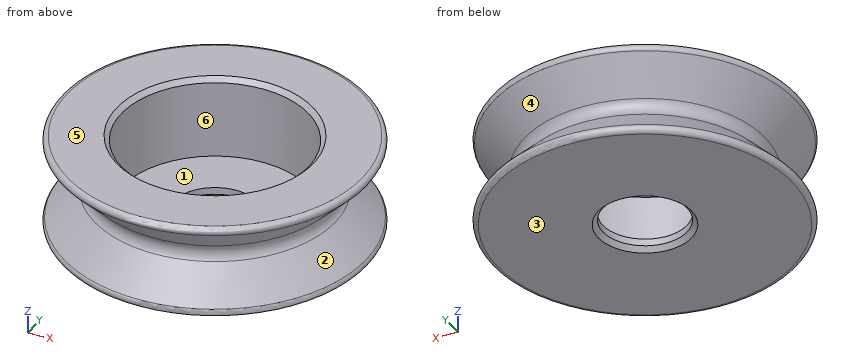
Solid Edge part; units mm, degrees
sketch "Sketch1" plane through (0, 0, 0) normal (0, -1, 0) x (1, 0, 0)
  line L0 (6.7929, 2) -> (1.8, 2)
  line L1 (1.8, 2) -> (1.8, -2)
  line L2 (1.8, -2) -> (6.7929, -2)
  line L3 (6.7929, -2) -> (5.1464, -0.3536)
  line L4 (5.1464, 0.3536) -> (6.7929, 2)
  arc A0 (5.1464, -0.3536) -> (5.1464, 0.3536) centre (5.5, 0) cw
revolve "RevolvedProtrusion1" add sketch "Sketch1" angle 360 about axis through (0, 0, 2) along (0, 0, -1)
fillet "Round1" radius 0.2 2 edges at (-6.7929, 0, 2) (-6.7929, 0, -2)
sketch "Sketch2" plane through (0, 0, 2) normal (0, 0, 1) x (0, 1, 0)
  circle A0 centre (0, 0) radius 4
extrude "VaciadoExtruido_2" cut sketch "Sketch2" against normal blind 3.5
chamfer "Chaflán_1" distance 0.2 angle 45 2 edges at (0, -4, 2) (-1.8, 0, -2)
Part model, mm, in its own coordinate system. Face numbers are marked on the shaded views. A direction names the side the tool comes from. Coordinates: 2 decimals unless noted, no trailing zeros. Order: outer loops, then holes, each group sorted by start corner. A loop starts at its lowest first (then second) coordinate and runs counter-clockwise, first axis right, second up. Notation, with made-up numbers: (20.5, 64) -> (65.5, 64) arc R15 ccw to (65.5, 81) -> close; hole circle Ø1 at (32.25, 45). An arc over 180 degrees is marked (long way). Put each result on its own line as item: value. Start each with the question number.
(1) Mould opens along Z. For the marked faces 1, 2, 3 and 4 say: pulls with the +Z half, pulls with the -Z half, needs draft (parallel to the pull), parting line crosses it, or undercut.
(2) Band-saw the part on C-C (z = 0.2). Give the cut face in (x, y).
(3) Band-saw the part on D-D (z = 1). Give the cut face in (x, y), then the cut area to 3 significant figures.
(4) Probe line 1 along X through (y, z) = (0, 1.15); line 2 along Y through (x, z) = (-0.25, 0.35); line 3 along Y through (x, z) = (-3.5, 1.4). List the from-to ranges inside material, lowest first. Write a range as [from, to].
(5) Band-saw the part on A-A (x = 0). Give the cut face in (y, z).
(6) Which spindle directions (+Z, -Z, +X, -X, +Y, -Y) get a long thin tool onto all of the face, cutting with end or side? Do the marked faces 5 and 6. Say none if no direction does.
(7) Pin check, flat tips, straight feed: pin 1 Ø4.5 at (x, y) = (0, 0) entering from +Z; pin 2 Ø1.5 at (y, z) = (-3.5, 1.5) entering from -X. Stop position of each tip, or through.
Determined:
1. face 1: pulls with the +Z half
1. face 2: undercut
1. face 3: pulls with the -Z half
1. face 4: undercut
2. outline: circle Ø10.08 at (0, 0); hole circle Ø8 at (0, 0)
3. outline: circle Ø11.59 at (0, 0); hole circle Ø8 at (0, 0)
3. area: 55.2 mm²
4. line 1: x = [-5.94, -4], [4, 5.94]
4. line 2: y = [-5.14, -3.99], [3.99, 5.14]
4. line 3: y = [-5.11, -1.94], [1.94, 5.11]
5. outline: (-6.45, -1.66) arc R0.2 ccw to (-6.31, -2) -> (-2, -2) -> (-1.8, -1.8) -> (-1.8, -1.5) -> (-4, -1.5) -> (-4, 1.8) -> (-4.2, 2) -> (-6.31, 2) arc R0.2 ccw to (-6.45, 1.66) -> (-5.15, 0.35) arc R0.5 cw to (-5.15, -0.35) -> close; (1.8, -1.8) -> (2, -2) -> (6.31, -2) arc R0.2 ccw to (6.45, -1.66) -> (5.15, -0.35) arc R0.5 cw to (5.15, 0.35) -> (6.45, 1.66) arc R0.2 ccw to (6.31, 2) -> (4.2, 2) -> (4, 1.8) -> (4, -1.5) -> (1.8, -1.5) -> close
6. face 5: +Z, +X, -X, +Y, -Y
6. face 6: +Z
7. pin 1: stops at z = -1.5
7. pin 2: stops at x = -5.87
